Autodesk Inventor part; units mm, degrees
ref_plane "YZ Plane" through (0, 0, 0) normal (1, 0, 0) x (0, 1, 0)
ref_plane "XZ Plane" through (0, 0, 0) normal (0, 1, 0) x (-1, 0, 0)
ref_plane "XY Plane" through (0, 0, 0) normal (0, 0, 1) x (1, 0, 0)
sketch "Sketch1" plane through (0, 0, 0) normal (0, 0, 1) x (1, 0, 0)
  line L0 (-25.4, -25.4) -> (25.4, -25.4)
  line L1 (25.4, -25.4) -> (25.4, 25.4)
  line L2 (25.4, 25.4) -> (-25.4, 25.4)
  line L3 (-25.4, 25.4) -> (-25.4, -25.4)
  line L4 (-25.4, -25.4) -> (25.4, 25.4) construction
  line L5 (25.4, -25.4) -> (-25.4, 25.4) construction
  line L6 (-22.225, 22.225) -> (22.225, 22.225)
  line L7 (22.225, 22.225) -> (22.225, -22.225)
  line L8 (22.225, -22.225) -> (-22.225, -22.225)
  line L9 (-22.225, -22.225) -> (-22.225, 22.225)
  point P0 (0, 0)
  dimension "width" = 50.8
  dimension "height" = 50.8
  dimension "thickness" = 3.175
extrude "Extrusion1" add sketch "Sketch1" along normal mid plane 101.6
sketch "Sketch2" plane through (25.4, -25.4, 50.8) normal (1, 0, 0) x (0, 0, -1)
  line L0 (101.6, 50.8) -> (101.6, 0) construction
  line L1 (101.6, 0) -> (0, 0) construction
  line L2 (0, 0) -> (0, 50.8) construction
  line L3 (0, 50.8) -> (101.6, 50.8) construction
  circle A0 centre (50.8, 25.4) radius 38.1 construction
  line L4 (36.2198, 60.5998) -> (65.3802, 60.5998) construction
  point P0 (15.6002, 39.9802)
  point P1 (15.6002, 10.8198)
  point P2 (36.2198, -9.7998)
  point P3 (65.3802, -9.7998)
  point P4 (85.9998, 10.8198)
  point P5 (85.9998, 39.9802)
  dimension "d5" = 76.2
  dimension "d8" = 360
hole "Hole1" at (25.4, 35.1998, -14.5802) at (25.4, 35.1998, 14.5802) at (25.4, 14.5802, 35.1998) at (25.4, -14.5802, 35.1998) at (25.4, -35.1998, 14.5802) at (25.4, -35.1998, -14.5802) at (25.4, -14.5802, -35.1998) at (25.4, 14.5802, -35.1998) direction (-1, 0, 0) diameter 5.1054 depth 3.175
properties part number "EL2-A-007" material "Aluminum 6061"
The listing builds one solid part. Answer for the finished solid, in the listing's coordinates (mm). A direction names the side the tool comes from. Coordinates: 2 decimals unless noted, no trailing zeros. Order: outer loops, then holes, each group sorted by start corner. A loop starts at its lowest first (then second) coordinate and runs counter-clockwise, first axis right, second up. Notation, with made-up numbers: M -3,69.25 L 42,69.25 A27 cw 42,85.25 Z; hole C 81,11.25 d7. An arc over 180 degrees is marked long. Answer as a JSON object with one key per item and string values. Group by question number.
1. Section B-B on x = -0.5 is taken. Write down the section's boundary in (y, z) (3 decimals).
2. Section D-D on z = -36 is taken. Write down the section's boundary in (x, y) (3 decimals), then the cut area to 3 significant figures.
3. Section A-A on z = 4 is taken. Write down the section's boundary in (x, y) (3 decimals).
4. Determine the mould class of faces 1 (the flat face through (-22.225, 0, -1)), 2 (the flat face through (-25.4, 0, -1)), 3 (the flat face through (0, -22.225, -1)), 4 (the cylindrical face through (23.79, 14.47, 37.75)) for opening direction X: released by +X, released by -X, zero draft, split by the parting line, or undercut.
5. A tool of negligible diameter and unlimited length cuts with its end or side. For faces 5 (the flat face through (22.225, 0, -1)), 6 (the flat face through (-23, 0, -50.8)), 7 (the cylindrical face through (23.79, 13.813, -37.635)), from which of +Z, -Z, +X, -X, +Y, -Y can it reach the whole face along a straight path? Write none if from no direction.
6. A straight line is drawn through the part: line 1 (X direction, y = -11, z = 27) (3 decimals). Find the intervals that lie inside material, in ascending order.
7. Flat-ended cylindrical pins translate along their axes: P1, Ø10, axis at x = -13, y = 12, coming from the -Z side; P2, Ø4.5, axis at y = -14.58, z = 35.2, coming from the +X side (3 decimals). Find the tip coordinate at first contact, or state that the pin passes through.
Values follow:
{
 "1": {"outline": "M -25.4,-50.8 L -22.225,-50.8 L -22.225,50.8 L -25.4,50.8 Z; M 22.225,-50.8 L 25.4,-50.8 L 25.4,50.8 L 22.225,50.8 Z"},
 "2": {"outline": "M -25.4,-25.4 L 25.4,-25.4 L 25.4,-17.004 L 22.225,-17.004 L 22.225,-22.225 L -22.225,-22.225 L -22.225,22.225 L 22.225,22.225 L 22.225,17.004 L 25.4,17.004 L 25.4,25.4 L -25.4,25.4 Z; M 22.225,-12.156 L 25.4,-12.156 L 25.4,12.156 L 22.225,12.156 Z", "area": "574 mm2"},
 "3": {"outline": "M -25.4,-25.4 L 25.4,-25.4 L 25.4,25.4 L -25.4,25.4 Z; hole M -22.225,-22.225 L 22.225,-22.225 L 22.225,22.225 L -22.225,22.225 Z"},
 "4": {"face 1": "undercut", "face 2": "released by -X", "face 3": "undercut", "face 4": "zero draft"},
 "5": {"face 5": "+Z, -Z", "face 6": "-Z, +X, -X, +Y, -Y", "face 7": "+X"},
 "6": {"line 1": "-25.4 to -22.225, 22.225 to 25.4"},
 "7": {"P1": "through", "P2": "x = -22.225"}
}
